```python
from build123d import *

# Parameters (mm, degrees)
SKETCH_1_R          = 2.1
EXTRUDE_1_DEPTH     = 4
SKETCH_2_R          = 1.6
CUT_EXTRUDE_1_DEPTH = 50


with BuildPart() as part:
    # 草图1 → 凸台-拉伸1 (new body)
    with BuildSketch(Plane(origin=(0, 0, 0), x_dir=(1, 0, 0), z_dir=(0, 1, 0))):
        Polygon((20, 0), (0, 0), (0, 45), (40.25, 85.25), (79.25, 85.25), (225.25, -60.75), (225.25, -99.75), (185, -140), (140, -140), (140, -120), (176.715728753, -120), (205.25, -91.465728753), (205.25, -69.034271247), (70.965728753, 65.25), (48.534271247, 65.25), (20, 36.715728753), align=None)
        with Locations(Location((10, 10, 0), (0, 0, 270))):
            Circle(SKETCH_1_R, mode=Mode.SUBTRACT)
        with Locations(Location((10, 35, 0), (0, 0, 90))):
            Circle(SKETCH_1_R, mode=Mode.SUBTRACT)
        with Locations(Location((175, -130, 0), (0, 0, 270))):
            Circle(SKETCH_1_R, mode=Mode.SUBTRACT)
        with Locations(Location((150, -130, 0), (0, 0, 90))):
            Circle(SKETCH_1_R, mode=Mode.SUBTRACT)
    extrude(amount=EXTRUDE_1_DEPTH)

    # 草图2 → 切除-拉伸1 (cut)
    with BuildSketch(Plane(origin=(0, 4, 0), x_dir=(1, 0, 0), z_dir=(0, 1, 0))):
        with Locations(Location((215.25, -94.75, 0), (0, 0, 270))):
            Circle(SKETCH_2_R)
        with Locations(Location((215.25, -74.75, 0), (0, 0, 270))):
            Circle(SKETCH_2_R)
        with Locations(Location((201.747474683, -51.389610307, 0), (0, 0, 270))):
            Circle(SKETCH_2_R)
        with Locations(Location((145.178932188, 5.178932188, 0), (0, 0, 270))):
            Circle(SKETCH_2_R)
        with Locations(Location((88.610389693, 61.747474683, 0), (0, 0, 90))):
            Circle(SKETCH_2_R)
        with Locations(Location((65.25, 75.25, 0), (0, 0, 90))):
            Circle(SKETCH_2_R)
        with Locations(Location((45.25, 75.25, 0), (0, 0, 90))):
            Circle(SKETCH_2_R)
    extrude(amount=-CUT_EXTRUDE_1_DEPTH, mode=Mode.SUBTRACT)


solid = part.part
```
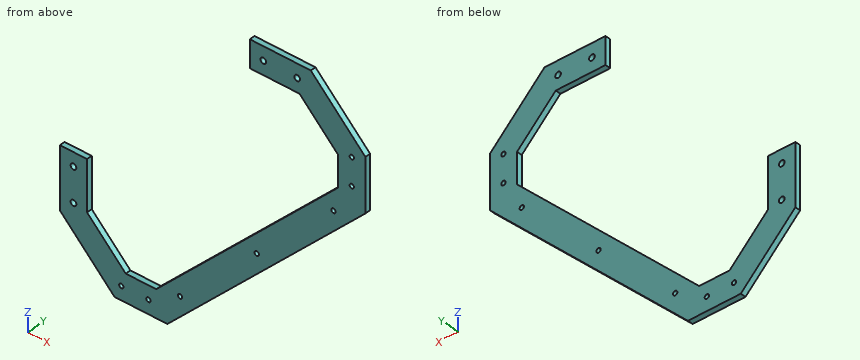
Source: CAD feature listing. Evaluate the final solid. Frame: model axes, mm. Round coordinates to 2 decimals unless told otherwise and drop trailing zeros. Order: outer loops, then holes, each group sorted by start corner. A loop starts at its lowest first (then second) coordinate and runs counter-clockwise, first axis right, second up. Notation, with made-up numbers: (75.5, 45.25) -> (85.5, 45.25) arc R19 ccw to (85.5, 52.25) -> close; hole circle Ø7 at (34, 37.25). An arc over 180 degrees is marked (long way). Use CSV: the item, a comma, the result in double quotes.
(1) Section A-A on x = 157. Return the cut outline in (y, z).
Report:
outline,"(0, -7.5) -> (4, -7.5) -> (4, 20.78) -> (0, 20.78) -> close; (0, 120) -> (4, 120) -> (4, 140) -> (0, 140) -> close"
(2) First-contact query: pin 1 Ø1.2 at (y, z) = (3, -15.5) entering from +X; pin 2 Ø1 at (x, y) = (91.5, 3) entering from +Z; pin 3 Ø2.5 at (x, z) = (10, -35) entering from -Y; pin 4 Ø2 at (y, z) = (3, 46) entering from +X. Flat tips, straight axial feed; report the tip coordinate or a pass-through.
Report:
pin 1,"x = 149.6"
pin 2,"z = -44.22"
pin 3,"through"
pin 4,"x = 211.5"
(3) Ray query, L1, parallel to X at y = 2.05, z = 129; L2, parallel to Z at x = 65.25, y = 3; L3, parallel to X at y = 2.8, z = -10. Return the intervals inside material, ascending.
Report:
L1,"140 to 148.15, 151.85 to 173.15, 176.85 to 196"
L2,"-85.25 to -76.85, -73.65 to -65.25"
L3,"0 to 7.9, 12.1 to 20, 126.22 to 154.5"
(4) Section C-C on x = 15. Return the cut outline in (y, z).
Report:
outline,"(0, -60) -> (4, -60) -> (4, 0) -> (0, 0) -> close"
(5) Section B-B on y = 1.5. Count the separate pieces of the cut face and the enclosed holes in it, and give its area (3 significant figures).
Report:
separate pieces,"1"
enclosed holes,"11"
area,"8,660 mm^2"
(6) Section D-D on z = 33. Return the cut outline in (x, y), and give its area (3 significant figures).
Report:
outline,"(169.22, 0) -> (197.5, 0) -> (197.5, 4) -> (169.22, 4) -> close"
area,"113 mm^2"
